```python
from build123d import *

# Parameters (mm, degrees)
PAD011_DEPTH    = 10
PAD012_DEPTH    = 4.8
SKETCH024_R     = 33.4
PAD013_DEPTH    = 3.2
POCKET007_DEPTH = 2.456658
POCKET008_DEPTH = 1.625221
SKETCH023_W     = 28
SKETCH023_H     = 9
POCKET009_DEPTH = 5
SKETCH022_R     = 3.4
POCKET010_DEPTH = 5
SKETCH025_R     = 0.8
POCKET011_DEPTH = 13.201


with BuildPart() as part:
    # CopySketch013 → Pad011 (new body)
    with BuildSketch(Plane.XY):
        with BuildLine():
            ThreePointArc((-34.481879, -6), (35, 0), (-34.481879, 6))
            Line((-34.481879, 6), (-34.481879, -6))
        make_face()
        with BuildLine():
            ThreePointArc((-27.36421, 15.4), (-29.127032, 11.729279), (-30.4, 7.861298))
            Line((-30.4, 7.861298), (-30.4, -7.861298))
            ThreePointArc((-30.4, -7.861298), (-29.127032, -11.729279), (-27.36421, -15.4))
            Line((-27.36421, -15.4), (-23, -15.4))
            ThreePointArc((-19.4, -18.999985), (-20.454421, -16.45441), (-23, -15.4))
            Line((-19.4, -18.999985), (-19.4, -24.690079))
            ThreePointArc((-19.4, -24.690079), (0, -31.4), (19.4, -24.690079))
            Line((19.4, -19), (19.4, -24.690079))
            ThreePointArc((23, -15.4), (20.454416, -16.454416), (19.4, -19))
            Line((23, -15.4), (27.36421, -15.4))
            ThreePointArc((27.36421, -15.4), (31.4, 0), (27.36421, 15.4))
            Line((23, 15.4), (27.36421, 15.4))
            ThreePointArc((19.4, 19), (20.454416, 16.454416), (23, 15.4))
            Line((19.4, 24.690079), (19.4, 19))
            ThreePointArc((19.4, 24.690079), (-0.385273, 31.397636), (-20, 24.206611))
            Line((-20, 24.206611), (-20, 17.010025))
            ThreePointArc((-23, 15.4), (-21.297635, 15.827942), (-20, 17.010025))
            Line((-23, 15.4), (-27.36421, 15.4))
        make_face(mode=Mode.SUBTRACT)
    extrude(amount=PAD011_DEPTH)

    # Sketch019 → Pad012 (join)
    with BuildSketch(Plane.XY):
        with BuildLine():
            ThreePointArc((-34.481879, -6), (35, 0), (-34.481879, 6))
            Line((-34.481879, 6), (-34.481879, -6))
        make_face()
        with BuildLine():
            ThreePointArc((-32.856658, -6), (33.4, 0), (-32.856658, 6))
            Line((-32.856658, 6), (-32.856658, -6))
        make_face(mode=Mode.SUBTRACT)
    extrude(amount=-PAD012_DEPTH)

    # Sketch024 → Pad013 (join)
    with BuildSketch(Plane.XY.offset(10)):
        with BuildLine():
            ThreePointArc((-34.481879, -6), (35, 0), (-34.481879, 6))
            Line((-34.481879, 6), (-34.481879, -6))
        make_face()
        Circle(SKETCH024_R, mode=Mode.SUBTRACT)
    extrude(amount=PAD013_DEPTH)

    # Sketch020 (on Face19 of Pad013) → Pocket007 (cut)
    with BuildSketch(Plane.YZ.offset(-30.4)):
        with BuildLine():
            ThreePointArc((-4, 3.68), (-5.414214, 3.094214), (-6, 1.68))
            Line((-6, 1.68), (-6, -3.6))
            Line((-6, -3.6), (6, -3.6))
            Line((6, 1.68), (6, -3.6))
            ThreePointArc((6, 1.68), (5.414214, 3.094214), (4, 3.68))
            Line((-4, 3.68), (4, 3.68))
        make_face()
    extrude(amount=-POCKET007_DEPTH, mode=Mode.SUBTRACT)

    # Sketch021 → Pocket008 (cut)
    with BuildSketch(Plane(origin=(-34.481879, 0, 0), x_dir=(0, -1, 0), z_dir=(-1, 0, 0))):
        with BuildLine():
            ThreePointArc((2.9, -0.32), (4.9, 1.68), (2.9, 3.68))
            Line((2.9, 3.68), (-2.9, 3.68))
            ThreePointArc((-2.9, 3.68), (-4.9, 1.68), (-2.9, -0.32))
            Line((2.9, -0.32), (-2.9, -0.32))
        make_face()
    extrude(amount=-POCKET008_DEPTH, mode=Mode.SUBTRACT)

    # Sketch023 → Pocket009 (cut)
    with BuildSketch(Plane.XZ.offset(31)):
        with Locations((0, 4.5)):
            Rectangle(SKETCH023_W, SKETCH023_H)
    extrude(amount=-POCKET009_DEPTH, mode=Mode.SUBTRACT)

    # Sketch022 → Pocket010 (cut)
    with BuildSketch(Plane.XZ.offset(35)):
        with Locations((-9.5, 4)):
            Circle(SKETCH022_R)
        with Locations((9.5, 4)):
            Circle(SKETCH022_R)
    extrude(amount=-POCKET010_DEPTH, mode=Mode.SUBTRACT)

    # Sketch025 → Pocket011 (cut, through all)
    with BuildSketch(Plane.XY):
        with Locations((-23, 19)):
            Circle(SKETCH025_R)
        with Locations((23, 19)):
            Circle(SKETCH025_R)
        with Locations((-23, -19)):
            Circle(SKETCH025_R)
        with Locations((23, -19)):
            Circle(SKETCH025_R)
    extrude(amount=POCKET011_DEPTH, mode=Mode.SUBTRACT)


solid = part.part
```
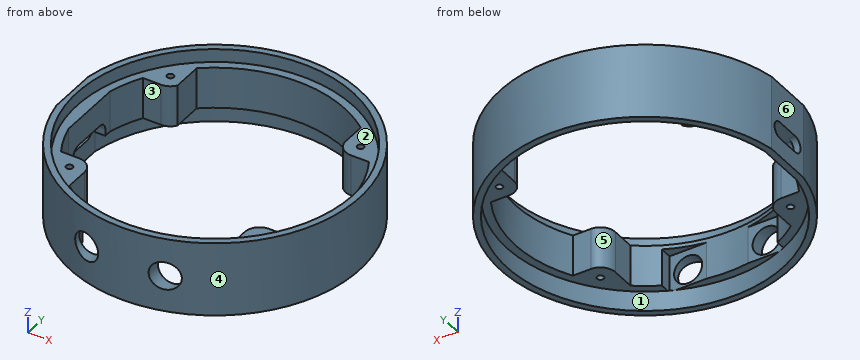
CAD build for the part. Positions are in the model's coordinates, mm. Face numbers are marked on the shaded views. A direction names the side the tool comes from. Give positions to 0.01 mm unless a question says otherwise; leave off trailing zeros. Loops run counter-clockwise (first coordinate to the right, second up) from the corner with the lowest first, then second, coordinate; pieces in that order, holes last. Notation, with made-up numbers: (20.25, -35.5) -> (49.25, -35.5) arc R22 cw to (49.25, -29.5) -> close; hole circle Ø6 at (67, -23.5). An arc over 180 degrees is marked (long way). Use a Markdown table: item, result.
1. Mould opens along Y. For the marked faces 4, 5 and 6 say: pulls with the +Y half, pulls with the -Y half, needs draft (parallel to the pull), parting line crosses it, or undercut.
Check result:
| item | result |
|---|---|
| face 4 | parting line crosses it |
| face 5 | undercut |
| face 6 | needs draft |
2. Slice it at D-D (x = -9.5). List the corners of the cut face in (y, z), plus the area to 3 significant figures.
Check result:
| item | result |
|---|---|
| outline | (-33.69, -4.8) -> (-32.02, -4.8) -> (-32.02, 0) -> (-31, 0) -> (-31, 0.6) -> (-33.69, 0.6) -> close; (-33.69, 7.4) -> (-31, 7.4) -> (-31, 9) -> (-29.93, 9) -> (-29.93, 10) -> (-32.02, 10) -> (-32.02, 13.2) -> (-33.69, 13.2) -> close; (29.93, 0) -> (32.02, 0) -> (32.02, -4.8) -> (33.69, -4.8) -> (33.69, 13.2) -> (32.02, 13.2) -> (32.02, 10) -> (29.93, 10) -> close |
| area | 73.9 mm^2 |
3. Slice it at B-B (y = 0). List the corners of the cut face in (x, z).
Check result:
| item | result |
|---|---|
| outline | (-34.48, -4.8) -> (-32.86, -4.8) -> (-32.86, -0.32) -> (-34.48, -0.32) -> close; (-34.48, 3.68) -> (-30.4, 3.68) -> (-30.4, 10) -> (-33.4, 10) -> (-33.4, 13.2) -> (-34.48, 13.2) -> close; (31.4, 0) -> (33.4, 0) -> (33.4, -4.8) -> (35, -4.8) -> (35, 13.2) -> (33.4, 13.2) -> (33.4, 10) -> (31.4, 10) -> close |
4. Which spindle directions (+Z, -Z, +X, -X, +Y, -Y) get a long thin tool onto all of the face, cutting with end or side? Do the marked faces 1, 2 and 3. Say none if no direction does.
Check result:
| item | result |
|---|---|
| face 1 | -Z |
| face 2 | +Z |
| face 3 | +Z, -Z |
5. Slice it at C-C (z = 6). Give the number of separate pieces and of enclosed holes in the cut face, plus the area to 3 significant figures.
Check result:
| item | result |
|---|---|
| separate pieces | 2 |
| enclosed holes | 4 |
| area | 851 mm^2 |
6. Flat gauge pins, fed straight in: pin 1 (5 mm diameter, centred on x = 25.5, z = 6, fed in from +Y); pin 2 (4 mm diameter, centred on x = -9.5, z = 4, fed in from +Y); pin 3 (0.5 mm diameter, centred on x = -31, z = 0.5, fed in from -Y); pin 4 (8 mm diameter, centred on y = 1.5, z = 3.5, fed in from +X). Where does each tip first touch, or does it go through?
Check result:
| item | result |
|---|---|
| pin 1 | stops at y = 26.38 |
| pin 2 | stops at y = 34.19 |
| pin 3 | stops at y = -16.72 |
| pin 4 | stops at x = 35 |
7. Wall check: L1, parallel to X at y = 18.5, z = 1.5; L2, parallel to X at y = 19, z = 5.5; L3, parallel to Y at x = -23, z = 4. Give the ranges that are in metal, low to high. Write a range as [from, to].
Check result:
| item | result |
|---|---|
| L1 | x = [-29.71, -23.62], [-22.38, -20], [19.43, 22.38], [23.62, 29.71] |
| L2 | x = [-29.39, -23.8], [-22.2, -20], [19.4, 22.2], [23.8, 29.39] |
| L3 | y = [-26.38, -19.8], [-18.2, -15.4], [15.4, 18.2], [19.8, 26.38] |
8. Slice it at A-A (x = 0). List the corners of the cut face in (y, z).
Check result:
| item | result |
|---|---|
| outline | (-35, -4.8) -> (-33.4, -4.8) -> (-33.4, 0) -> (-31.4, 0) -> (-31.4, 10) -> (-33.4, 10) -> (-33.4, 13.2) -> (-35, 13.2) -> close; (31.4, 0) -> (33.4, 0) -> (33.4, -4.8) -> (35, -4.8) -> (35, 13.2) -> (33.4, 13.2) -> (33.4, 10) -> (31.4, 10) -> close |
